from build123d import *

# Parameters (mm, degrees)
SKETCH1_W           = 1117.6
SKETCH1_H           = 2162.175
BOSS_EXTRUDE1_DEPTH = 25.4
BOSS_EXTRUDE4_DEPTH = 21.59
SKETCH7_W           = 1117.6
SKETCH7_H           = 2162.175
BOSS_EXTRUDE5_DEPTH = 25.4
SKETCH8_W           = 1016
SKETCH8_H           = 2111.375
CUT_EXTRUDE2_DEPTH  = 2436.009405059
FILLET1_R           = 5.08


with BuildPart() as part:
    # Sketch1 → Boss-Extrude1 (new body)
    with BuildSketch(Plane.XY):
        with Locations((558.8, 1081.0875)):
            Rectangle(SKETCH1_W, SKETCH1_H)
    extrude(amount=BOSS_EXTRUDE1_DEPTH)

    # Sketch6 → Boss-Extrude4 (add)
    with BuildSketch(Plane(origin=(0, 0, 0), x_dir=(-1, 0, 0), z_dir=(0, 0, -1))):
        Polygon((-1066.8, 0), (-1092.2, 0), (-1092.2, 2136.775), (-25.4, 2136.775), (-25.4, 0), (-50.8, 0), (-50.8, 2111.375), (-1066.8, 2111.375), align=None)
    extrude(amount=BOSS_EXTRUDE4_DEPTH)

    # Sketch7 → Boss-Extrude5 (add)
    with BuildSketch(Plane(origin=(0, 0, -21.59), x_dir=(-1, 0, 0), z_dir=(0, 0, -1))):
        with Locations((-558.8, 1081.0875)):
            Rectangle(SKETCH7_W, SKETCH7_H)
    extrude(amount=BOSS_EXTRUDE5_DEPTH)

    # Sketch8 → Cut-Extrude2 (cut, through all)
    with BuildSketch(Plane.XY.offset(25.4)):
        with Locations((558.8, 1055.6875)):
            Rectangle(SKETCH8_W, SKETCH8_H)
    extrude(amount=-CUT_EXTRUDE2_DEPTH, mode=Mode.SUBTRACT)

    # Fillet1
    fillet1_edges = [part.edges().sort_by_distance(p)[0] for p in [
        (1117.6, 1081.0875, 25.4),
        (558.8, 2162.175, 25.4),
        (1117.6, 1081.0875, -46.99),
        (1092.2, 0, -46.99),
        (0, 1081.0875, -46.99),
        (558.8, 2162.175, -46.99),
        (0, 1081.0875, 25.4),
        (25.4, 0, -46.99),
        (1092.2, 0, 25.4),
        (50.8, 1055.6875, -46.99),
        (558.8, 2111.375, -46.99),
        (1066.8, 1055.6875, -46.99),
        (50.8, 1055.6875, 25.4),
        (1066.8, 1055.6875, 25.4),
        (558.8, 2111.375, 25.4),
        (25.4, 0, 25.4),
    ]]
    fillet(fillet1_edges, radius=FILLET1_R)


solid = part.part
The model under review builds one solid part; all positions refer to its coordinate system, in mm. A direction names the side the tool comes from. Give positions to 0.01 mm unless a question says otherwise; leave off trailing zeros. Order: outer loops, then holes, each group sorted by start corner. A loop starts at its lowest first (then second) coordinate and runs counter-clockwise, first axis right, second up. Notation, with made-up numbers: M 86,83 L 115,83 A26 cw 115,119 Z; hole C 70.5,-18.5 d11. An arc over 180 degrees is marked long. One line per question, with ' | ' between items. Start each with the question number.
1) Mouldability with a two-part tool opening along Z and no side actions: class faces 3 (the face through (1087, 0, -10)), 4 (the face through (1100, 1086, -21.59)), 5 (the face through (1089, 1405, 25.4)) as pulls with the +Z half, pulls with the -Z half, needs draft (parallel to the pull), parting line crosses it, or undercut.
2) Clearance check with flat-ended pins moving along their axes: P1, Ø6, axis at x = 496, z = -15, coming from the -Y side (3 decimals); P2, Ø11, axis at y = 827, z = -13, coming from the +X side; P3, Ø6.5, axis at y = 1099.5, z = -7.5, coming from the -X side; P4, Ø17.5, axis at x = 501, z = -6, coming from the +Y side (3 decimals). State where each tip first meets the part, or that it passes through.
3) Consider section B-B, the plane x = 440.5. Give the boundary of the cut face in (y, z) (3 decimals).
4) Wall thickness on L1, parallel to X at y = 1774.5, z = -7.5; L2, parallel to X at y = 1708, z = 7.5; L3, parallel to Y at x = 722, z = -27 (3 decimals): over which ranges is each line inside the solid? List them lowest first. Write a range as from..to.
5) Consider section A-A, the plane y = 1768. Give the boundary of the cut face in (x, z), then the cut area to 3 significant figures.
6) For faces 1 (the face through (1066.8, 1041, -10)), 2 (the face through (26, 0, -10)), list the 3-axis set-ups (+Z, -Z, +X, -X, +Y, -Y) from which the entire face can be reached by the end or side of a thin tool; tool diameter is ignored.
Found:
1) face 3: needs draft | face 4: undercut | face 5: pulls with the +Z half
2) P1: stops at y = 2111.375 | P2: stops at x = 1092.2 | P3: stops at x = 25.4 | P4: stops at y = 2162.175
3) outline: M 2111.375,-41.91 A5.08 ccw 2116.455,-46.99 L 2157.095,-46.99 A5.08 ccw 2162.175,-41.91 L 2162.175,-21.59 L 2136.775,-21.59 L 2136.775,0 L 2162.175,0 L 2162.175,20.32 A5.08 ccw 2157.095,25.4 L 2116.455,25.4 A5.08 ccw 2111.375,20.32 Z
4) L1: x = 25.4..50.8, 1066.8..1092.2 | L2: x = 0..50.8, 1066.8..1117.6 | L3: y = 2111.375..2162.175
5) outline: M 0,-41.91 A5.08 ccw 5.08,-46.99 L 45.72,-46.99 A5.08 ccw 50.8,-41.91 L 50.8,20.32 A5.08 ccw 45.72,25.4 L 5.08,25.4 A5.08 ccw 0,20.32 L 0,0 L 25.4,0 L 25.4,-21.59 L 0,-21.59 Z; M 1066.8,-41.91 A5.08 ccw 1071.88,-46.99 L 1112.52,-46.99 A5.08 ccw 1117.6,-41.91 L 1117.6,-21.59 L 1092.2,-21.59 L 1092.2,0 L 1117.6,0 L 1117.6,20.32 A5.08 ccw 1112.52,25.4 L 1071.88,25.4 A5.08 ccw 1066.8,20.32 Z | area: 6,210 mm²
6) face 1: +Z, -Z, -Y | face 2: +Z, -Z, +X, -X, -Y
